Input: part model. Units: mm. Frame: model coordinates. Coordinates: 2 decimals unless noted, no trailing zeros. Write each loop counter-clockwise with the first axis right and the second up, starting at its lowest first coordinate (ties: lowest second). Pieces come first, ordered by that corner, then holes. Notation, with made-up numbers: M -29,-21.75 L 11,-21.75 A12 ccw 11,-5.75 Z; hole C 4.5,37 d4. An arc over 180 degrees is marked long. Use CSV: the item, a comma, the result in double quotes.
```python
from build123d import *

# Parameters (mm, degrees)
SKETCH1_W           = 300
SKETCH1_H           = 11
SKETCH1_R           = 1.5
BOSS_EXTRUDE2_DEPTH = 4


with BuildPart() as part:
    # Sketch1 → Boss-Extrude2 (new body)
    with BuildSketch(Plane(origin=(0, 0, 0), x_dir=(1, 0, 0), z_dir=(0, 1, 0))):
        Rectangle(SKETCH1_W, SKETCH1_H)
        Circle(SKETCH1_R, mode=Mode.SUBTRACT)
        with BuildLine():
            Line((20, 1.5), (140, 1.5))
            ThreePointArc((140, 1.5), (141.5, 0), (140, -1.5))
            Line((140, -1.5), (20, -1.5))
            ThreePointArc((20, -1.5), (18.5, 0), (20, 1.5))
        make_face(mode=Mode.SUBTRACT)
        with BuildLine():
            Line((-20, -1.5), (-140, -1.5))
            ThreePointArc((-140, -1.5), (-141.5, 0), (-140, 1.5))
            Line((-140, 1.5), (-20, 1.5))
            ThreePointArc((-20, 1.5), (-18.5, 0), (-20, -1.5))
        make_face(mode=Mode.SUBTRACT)
    extrude(amount=BOSS_EXTRUDE2_DEPTH)


solid = part.part
```
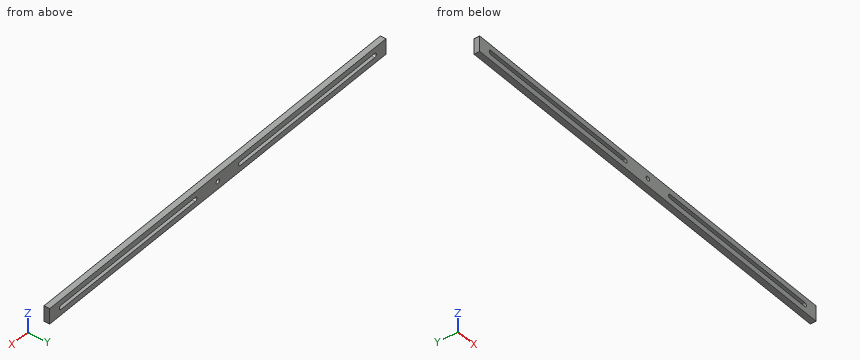
1. Section B-B (y = 3.1). Return loops of the section in (x, z).
Resolved:
outline,"M -150,-5.5 L 150,-5.5 L 150,5.5 L -150,5.5 Z; hole M -140,-1.5 L -20,-1.5 A1.5 ccw -20,1.5 L -140,1.5 A1.5 ccw Z; hole C 0,0 d3; hole M 20,-1.5 L 140,-1.5 A1.5 ccw 140,1.5 L 20,1.5 A1.5 ccw Z"
2. Material intervals for line 1 (X direction, y = 0.2, z = 0); line 2 (Z direction, x = 0, y = 1.35); line 3 (X direction, y = 2.9, z = 1.25), sorted ascending. Write a range as [from, to].
Resolved:
line 1,"x = [-150, -141.5], [-18.5, -1.5], [1.5, 18.5], [141.5, 150]"
line 2,"z = [-5.5, -1.5], [1.5, 5.5]"
line 3,"x = [-150, -140.83], [-19.17, -0.83], [0.83, 19.17], [140.83, 150]"
3. Section A-A (x = -71). Return loops of the section in (y, z).
Resolved:
outline,"M 0,-5.5 L 4,-5.5 L 4,-1.5 L 0,-1.5 Z; M 0,1.5 L 4,1.5 L 4,5.5 L 0,5.5 Z"
